from build123d import *

# Parameters (mm, degrees)
F0_W     = 152.4
F0_H     = 127
F1_DEPTH = 76.2
F2_W     = 127
F2_H     = 101.6
F3_DEPTH = 50.8
F4_R     = 5.08


with BuildPart() as f1:
    # F0 (on Front) → F1 (new body)
    with BuildSketch(Plane.XZ):
        Rectangle(F0_W, F0_H)
    extrude(amount=-F1_DEPTH)

    # F2 (on face) → F3 (cut)
    with BuildSketch(Plane.XZ):
        Rectangle(F2_W, F2_H)
    extrude(amount=-F3_DEPTH, mode=Mode.SUBTRACT)

    # F4
    f4_edges = [f1.edges().sort_by_distance(p)[0] for p in [
        (0, 0, 50.8),
        (0, 0, 63.5),
        (63.5, 0, 0),
        (0, 0, -50.8),
        (-63.5, 0, 0),
        (-76.2, 0, 0),
        (0, 0, -63.5),
        (76.2, 0, 0),
    ]]
    fillet(f4_edges, radius=F4_R)


solid = f1.part
Work out the finished part from the listing and answer in its coordinate system (mm). A direction names the side the tool comes from. Give positions to 0.01 mm unless a question says otherwise; leave off trailing zeros. Order: outer loops, then holes, each group sorted by start corner. A loop starts at its lowest first (then second) coordinate and runs counter-clockwise, first axis right, second up. Notation, with made-up numbers: (4, -5) - (30, -5) arc R13 ccw to (30, 10) - close; hole circle Ø4 at (-19, 67). An arc over 180 degrees is marked (long way). Answer as CSV lines item,"result". Start each with the question number.
Q1. The mould has two halves that part along X. Classify faces 3 (the face through (0.96, 1.449, 52.328)), 4 (the face through (76.2, 40, -1)), 5 (the face through (-76.2, 40, -1)): +X half, -X half, draft (parallel to the pull), parting line (faces both ways), or undercut.
Q2. Find the intervals of material crossed by L1, parallel to X at y = 9, z = 43.5; L2, parallel to Z at x = 59, y = 47; L3, parallel to Y at x = -31.5, z = -20.5, in increasing order. Write a range as [from, to].
Q3. Given pin 1 Ø5 at (x, z) = (-11, -27.5) entering from -Y, flat-ended and moving along its own axis, determine where the tip first touches the part or whether it passes through.
Q4. The part is cut by section C-C (z = -46). Write down the section's boundary in (x, y), then the cut area to 3 significant figures.
Q5. The part is cut by section B-B (x = 20.5). Write down the section's boundary in (y, z), then the cut area to 3 significant figures.
Q6. For faces 1 (the face through (1.067, 1.528, -62.051)), 2 (the face through (0.96, 1.449, -52.328)), determine the directions among +Z, -Z, +X, -X, +Y, -Y from which every point of the face is accessible in a straight line to the end or side of a thin tool.
Q7. The part is cut by section A-A (y = 18). Write down the section's boundary in (x, z).
Check result:
1,face 3,"undercut"
1,face 4,"+X half"
1,face 5,"-X half"
2,L1,"x = [-76.2, -63.5], [63.5, 76.2]"
2,L2,"z = [-63.5, -50.8], [50.8, 63.5]"
2,L3,"y = [50.8, 76.2]"
3,pin 1,"stops at y = 50.8"
4,outline,"(-76.2, 5.08) arc R5.08 ccw to (-71.12, 0) - (-68.58, 0) arc R5.08 ccw to (-63.5, 5.08) - (-63.5, 50.8) - (63.5, 50.8) - (63.5, 5.08) arc R5.08 ccw to (68.58, 0) - (71.12, 0) arc R5.08 ccw to (76.2, 5.08) - (76.2, 76.2) - (-76.2, 76.2) - close"
4,area,"5,140 mm²"
5,outline,"(0, -58.42) arc R5.08 ccw to (5.08, -63.5) - (76.2, -63.5) - (76.2, 63.5) - (5.08, 63.5) arc R5.08 ccw to (0, 58.42) - (0, 55.88) arc R5.08 ccw to (5.08, 50.8) - (50.8, 50.8) - (50.8, -50.8) - (5.08, -50.8) arc R5.08 ccw to (0, -55.88) - close"
5,area,"4,490 mm²"
6,face 1,"-Z, +X, -X, -Y"
6,face 2,"-Y"
7,outline,"(-76.2, -63.5) - (76.2, -63.5) - (76.2, 63.5) - (-76.2, 63.5) - close; hole (-63.5, -50.8) - (63.5, -50.8) - (63.5, 50.8) - (-63.5, 50.8) - close"
